from build123d import *

# Parameters (mm, degrees)
SKETCH2_W           = 170
SKETCH2_H           = 130
BOSS_EXTRUDE1_DEPTH = 3
SKETCH3_R           = 1.5
CUT_EXTRUDE1_DEPTH  = 108.046718773
SKETCH4_R           = 1.75
SKETCH4_R_2         = 1.5
SKETCH4_R_3         = 1.85
CUT_EXTRUDE2_DEPTH  = 108.046718773
FILLET1_R           = 15


with BuildPart() as part:
    # Sketch2 → Boss-Extrude1 (new body)
    with BuildSketch(Plane(origin=(0, 0, 0), x_dir=(1, 0, 0), z_dir=(0, 1, 0))):
        Rectangle(SKETCH2_W, SKETCH2_H)
    extrude(amount=BOSS_EXTRUDE1_DEPTH)

    # Sketch3 → Cut-Extrude1 (cut, through all)
    with BuildSketch(Plane.XZ):
        with Locations(Location((32.25, 57.816706978, 0), (0, 0, 270))):
            Circle(SKETCH3_R)
        with Locations(Location((-32.25, -57.816706978, 0), (0, 0, 270))):
            Circle(SKETCH3_R)
        with Locations(Location((-32.25, 57.816706978, 0), (0, 0, 270))):
            Circle(SKETCH3_R)
        with Locations(Location((32.25, -57.816706978, 0), (0, 0, 270))):
            Circle(SKETCH3_R)
    extrude(amount=-CUT_EXTRUDE1_DEPTH, mode=Mode.SUBTRACT)

    # Sketch4 → Cut-Extrude2 (cut, through all)
    with BuildSketch(Plane(origin=(0, 3, 0), x_dir=(1, 0, 0), z_dir=(0, 1, 0))):
        with Locations(Location((13.7, 27.2, 0), (0, 0, 270))):
            Circle(SKETCH4_R)
        with Locations(Location((-21.7, 45.8, 0), (0, 0, 270))):
            Circle(SKETCH4_R)
        with Locations(Location((-10.5, -26.5, 0), (0, 0, 270))):
            Circle(SKETCH4_R_2)
        with Locations(Location((10.5, -26.5, 0), (0, 0, 270))):
            Circle(SKETCH4_R_2)
        with Locations(Location((10.5, -57.5, 0), (0, 0, 270))):
            Circle(SKETCH4_R_2)
        with Locations(Location((-10.5, -57.5, 0), (0, 0, 270))):
            Circle(SKETCH4_R_2)
        with Locations(Location((76.6, -10.9, 0), (0, 0, 270))):
            Circle(SKETCH4_R_3)
        with Locations(Location((76.6, -47.6, 0), (0, 0, 270))):
            Circle(SKETCH4_R_3)
        with Locations(Location((39.9, -47.6, 0), (0, 0, 270))):
            Circle(SKETCH4_R_3)
        with Locations(Location((39.9, -10.9, 0), (0, 0, 270))):
            Circle(SKETCH4_R_3)
        with Locations(Location((39.9, 47.6, 0), (0, 0, 270))):
            Circle(SKETCH4_R_3)
        with Locations(Location((76.6, 47.6, 0), (0, 0, 270))):
            Circle(SKETCH4_R_3)
        with Locations(Location((76.6, 10.9, 0), (0, 0, 270))):
            Circle(SKETCH4_R_3)
        with Locations(Location((39.9, 10.9, 0), (0, 0, 270))):
            Circle(SKETCH4_R_3)
        with Locations(Location((4.5, -10.5, 0), (0, 0, 270))):
            Circle(SKETCH4_R_2)
        with Locations(Location((4.5, 10.5, 0), (0, 0, 270))):
            Circle(SKETCH4_R_2)
    extrude(amount=-CUT_EXTRUDE2_DEPTH, mode=Mode.SUBTRACT)

    # Fillet1
    fillet1_edges = [part.edges().sort_by_distance(p)[0] for p in [
        (85, 1.5, 65),
        (-85, 1.5, 65),
        (-85, 1.5, -65),
        (85, 1.5, -65),
    ]]
    fillet(fillet1_edges, radius=FILLET1_R)


solid = part.part
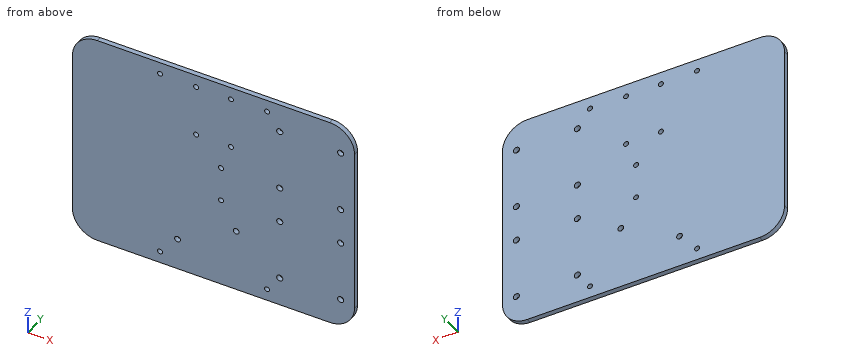
Work out the finished part from the listing and answer in its coordinate system (mm). Round coordinates to 2 decimals unless told otherwise and drop trailing zeros. Order: outer loops, then holes, each group sorted by start corner. A loop starts at its lowest first (then second) coordinate and runs counter-clockwise, first axis right, second up. Notation, with made-up numbers: M 29.5,-30 L 53.5,-30 A20 ccw 53.5,6 Z; hole C 23.5,52 d9. An arc over 180 degrees is marked long. Put each result on its own line as item: value. Start each with the question number.
Q1. Section A-A, the plane x = 39.9 is taken. Write down the section's boundary in (y, z), and give its area (3 significant figures).
Q2. A flat-ended cylindrical pin translates along its axis: pin 1 (2.5 mm diameter, centred on x = -32.25, z = 57.82, fed in from -Y). Find the tip coordinate at first contact, or state that the pin passes through.
Q3. Straight lines are drawn through the part: L1, parallel to X at y = 2.25, z = 26.5; L2, parallel to X at y = 1.9, z = 47.6; L3, parallel to Z at x = 32, y = 1.8. For each, find the intervals that lie inside material, in ascending order. Write a range as [from, to].
Q4. Section B-B, the plane y = 0.65 is taken. Give the number of separate pieces and of enclosed holes in the cut face, and give its area (3 significant figures).
Findings below:
1. outline: M 0,-65 L 3,-65 L 3,-49.45 L 0,-49.45 Z; M 0,-45.75 L 3,-45.75 L 3,-12.75 L 0,-12.75 Z; M 0,-9.05 L 3,-9.05 L 3,9.05 L 0,9.05 Z; M 0,12.75 L 3,12.75 L 3,45.75 L 0,45.75 Z; M 0,49.45 L 3,49.45 L 3,65 L 0,65 Z
1. area: 346 mm^2
2. pin 1: passes through
3. L1: x = [-85, -12], [-9, 9], [12, 85]
3. L2: x = [-85, 38.05], [41.75, 74.75], [78.45, 85]
3. L3: z = [-65, -59.3], [-56.34, 56.34], [59.3, 65]
4. separate pieces: 1
4. enclosed holes: 20
4. area: 21,700 mm^2
